Check sheet for the modelled part. Datum: model origin and axes. Units: mm. A direction names the side the tool comes from. Give positions to 0.01 mm unless a question says otherwise; leave off trailing zeros. Order: outer loops, then holes, each group sorted by start corner. A loop starts at its lowest first (then second) coordinate and runs counter-clockwise, first axis right, second up. Notation, with made-up numbers: (-7, -11.75) -> (44, -11.75) arc R33 cw to (44, 21.25) -> close; hole circle Ø8 at (-21, 30.5). An arc over 180 degrees is marked (long way). Answer in a Markdown table with one row per item. Add a question column.
(1) Thickness scan on L1, parallel to Y at x = 25.4, z = 3.25 (3 decimals); L2, parallel to X at y = 14.5, z = 6.75; L3, parallel to X at y = -15.5, z = 8.75. Record the ranges inside material, lowest first. Write a range as [from, to].
(2) Cross-section at B-B (y = 11). Record the cut outline in (x, z).
(3) Cross-section at C-C (x = -2.5). Record the cut outline in (y, z).
(4) Cross-section at A-A (z = 5). Record the cut outline in (x, y) (3 decimals), then the cut area to 3 significant figures.
(5) Set-up check for faces 1 (the face through (23, 9.525, 5)), 2 (the face through (-0.121, -19.193, 4.93)): record each of +Z, -Z, +X, -X, +Y, -Y from which the full face is reachable in a straight line by a thin tool's end or side.
(6) Go/stop test with flat-tipped pins: pin 1 (3 mm diameter, centred on x = 25.4, y = -14.75, fed in from -Z); pin 2 (2 mm diameter, centred on y = -11.5, z = 4, fed in from +X); pin 3 (4 mm diameter, centred on x = 6.5, z = 1, fed in from +Y); pin 4 (1.5 mm diameter, centred on y = -13.5, z = 3, fed in from -X). Record where each tip stops, or that it passes through.
(7) Release check for a two-part mould opening along X. For faces 3 (the face through (19.193, -0.088, 4.93)), 4 (the face through (17, -19.975, 5)), 5 (the face through (25.01, -16.507, 4.93)) record: released by +X, released by -X, zero draft, split by the parting line, or undercut.
```python
from build123d import *

# Parameters (mm, degrees)
SKETCH1_R           = 1.8
BOSS_EXTRUDE1_DEPTH = 10


with BuildPart() as part:
    # Sketch1 → Boss-Extrude1 (new body)
    with BuildSketch(Plane.XY):
        with BuildLine():
            Line((8.562572408, -19.9749896), (25.4, -19.9749896))
            ThreePointArc((25.4, -19.9749896), (30.6249948, -14.7499948), (25.4, -9.525))
            Line((25.4, -9.525), (20.579786947, -9.525))
            ThreePointArc((20.579786947, -9.525), (18.515185258, -8.464533666), (18.174552534, -6.168637692))
            ThreePointArc((18.174552534, -6.168637692), (19.192875, 0), (18.174552534, 6.168637692))
            ThreePointArc((18.174552534, 6.168637692), (18.515185258, 8.464533666), (20.579786947, 9.525))
            Line((20.579786947, 9.525), (25.4, 9.525))
            ThreePointArc((25.4, 9.525), (30.6249948, 14.7499948), (25.4, 19.9749896))
            Line((25.4, 19.9749896), (8.562572408, 19.9749896))
            ThreePointArc((8.562572408, 19.9749896), (0, 19.192875), (-8.562572408, 19.9749896))
            Line((-8.562572408, 19.9749896), (-25.4, 19.9749896))
            ThreePointArc((-25.4, 19.9749896), (-30.6249948, 14.7499948), (-25.4, 9.525))
            Line((-25.4, 9.525), (-20.579786947, 9.525))
            ThreePointArc((-20.579786947, 9.525), (-18.515185258, 8.464533666), (-18.174552534, 6.168637692))
            ThreePointArc((-18.174552534, 6.168637692), (-19.192875, 0), (-18.174552534, -6.168637692))
            ThreePointArc((-18.174552534, -6.168637692), (-18.515185258, -8.464533666), (-20.579786947, -9.525))
            Line((-20.579786947, -9.525), (-25.4, -9.525))
            ThreePointArc((-25.4, -9.525), (-30.6249948, -14.7499948), (-25.4, -19.9749896))
            Line((-25.4, -19.9749896), (-8.562572408, -19.9749896))
            ThreePointArc((-8.562572408, -19.9749896), (0, -19.192875), (8.562572408, -19.9749896))
        make_face()
        with Locations((-25.4, 14.7499948)):
            Circle(SKETCH1_R, mode=Mode.SUBTRACT)
        with Locations((-25.4, -14.7499948)):
            Circle(SKETCH1_R, mode=Mode.SUBTRACT)
        with Locations((25.4, -14.7499948)):
            Circle(SKETCH1_R, mode=Mode.SUBTRACT)
        with Locations((25.4, 14.7499948)):
            Circle(SKETCH1_R, mode=Mode.SUBTRACT)
    extrude(amount=BOSS_EXTRUDE1_DEPTH)


solid = part.part
```
Answer below:
| question | item | result |
|---|---|---|
| 1 | L1 | y = [-19.975, -16.55], [-12.95, -9.525], [9.525, 12.95], [16.55, 19.975] |
| 1 | L2 | x = [-30.62, -27.18], [-23.62, 23.62], [27.18, 30.62] |
| 1 | L3 | x = [-30.57, -27.04], [-23.76, 23.76], [27.04, 30.57] |
| 2 | outline | (-29.04, 0) -> (29.04, 0) -> (29.04, 10) -> (-29.04, 10) -> close |
| 3 | outline | (-19.26, 0) -> (19.26, 0) -> (19.26, 10) -> (-19.26, 10) -> close |
| 4 | outline | (-25.4, -19.975) -> (-8.563, -19.975) arc R47.262 cw to (8.563, -19.975) -> (25.4, -19.975) arc R5.225 ccw to (25.4, -9.525) -> (20.58, -9.525) arc R2.54 cw to (18.175, -6.169) arc R19.193 ccw to (18.175, 6.169) arc R2.54 cw to (20.58, 9.525) -> (25.4, 9.525) arc R5.225 ccw to (25.4, 19.975) -> (8.563, 19.975) arc R47.262 cw to (-8.563, 19.975) -> (-25.4, 19.975) arc R5.225 ccw to (-25.4, 9.525) -> (-20.58, 9.525) arc R2.54 cw to (-18.175, 6.169) arc R19.193 ccw to (-18.175, -6.169) arc R2.54 cw to (-20.58, -9.525) -> (-25.4, -9.525) arc R5.225 ccw to start; hole circle Ø3.6 at (-25.4, -14.75); hole circle Ø3.6 at (-25.4, 14.75); hole circle Ø3.6 at (25.4, -14.75); hole circle Ø3.6 at (25.4, 14.75) |
| 4 | area | 1,890 mm² |
| 5 | face 1 | +Z, -Z, +X |
| 5 | face 2 | +Z, -Z, -Y |
| 6 | pin 1 | passes through |
| 6 | pin 2 | stops at x = 30.12 |
| 6 | pin 3 | stops at y = 19.96 |
| 6 | pin 4 | stops at x = -30.6 |
| 7 | face 3 | released by +X |
| 7 | face 4 | zero draft |
| 7 | face 5 | undercut |
